Verification items for this drawing (mm, ordinates from the low corner). A direction names the side the tool comes from. Round coordinates to 2 decimals unless told otherwise and drop trailing zeros. Loops run counter-clockwise (first coordinate to the right, second up) from the corner with the lowest first, then second, coordinate; pieces in that order, holes last. Notation, with made-up numbers: (20, -7) - (36, -7) arc R10 ccw to (36, 12) - close; hole circle Ø10 at (59.25, 77). An arc over 180 degrees is marked (long way). Use a Markdown table: item, result. Add a question column.
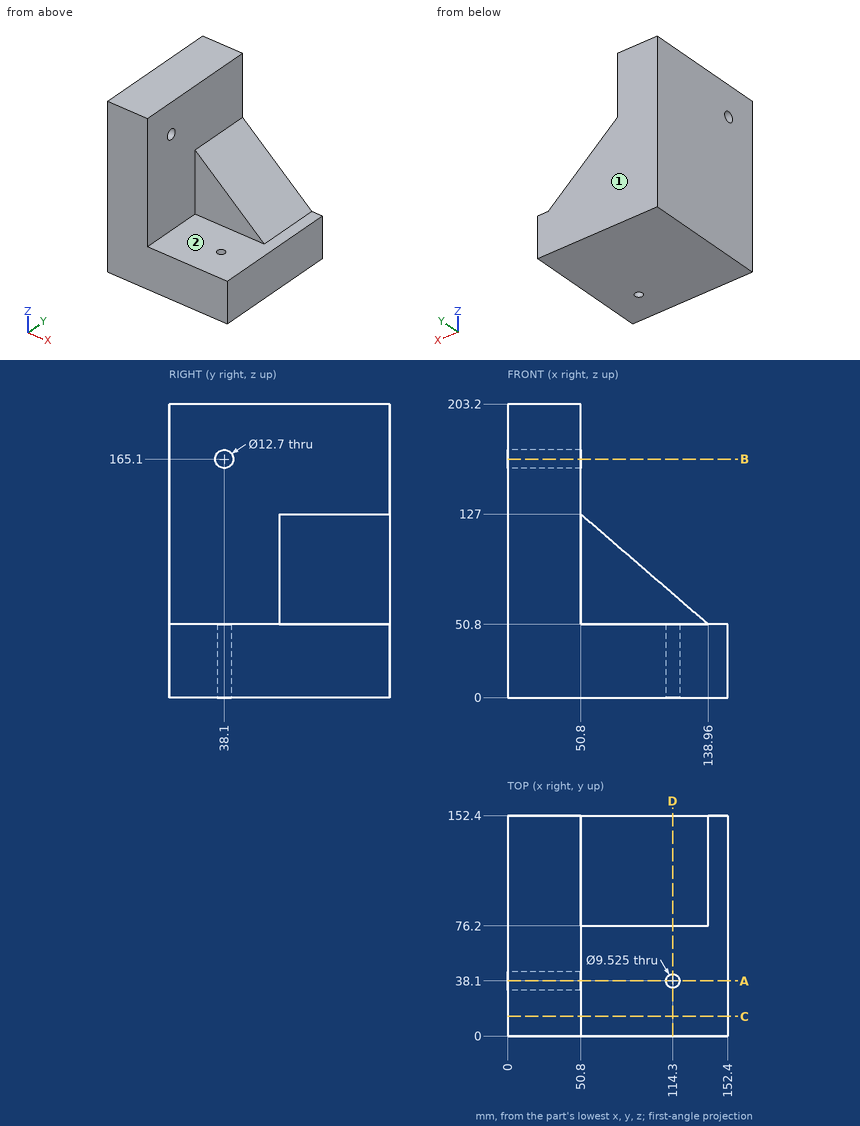
Q1. Section check D-D on x = 114.3. Record the cut outline in (y, z), plus the area to 3 significant figures.
Q2. Go/stop test with flat-tipped pins: pin 1 Ø5 at (y, z) = (36.5, 58.5) entering from +X; pin 2 Ø3 at (x, z) = (98.5, 77.5) entering from -Y. Record where each tip stops, or that it passes through.
Q3. Section check B-B on z = 165.1. Record the cut outline in (x, y).
Q4. Thickness scan on line 1 along Y through (x, z) = (18, 165); line 2 along Z through (x, y) = (31, 38); line 3 along Y through (x, z) = (114.3, 26.5). Record the ranges inside material, lowest first.
Q5. Section check C-C on y = 13.5. Record the cut outline in (x, z).
Q6. Set-up check for the marked faces 1 and 2: record each of +Z, -Z, +X, -X, +Y, -Y from which the full face is reachable in a straight line by a thin tool's end or side.
Q7. Section check A-A on y = 38.1. Record the cut outline in (x, z).
Determined:
| question | item | result |
|---|---|---|
| 1 | outline | (0, 0) - (33.34, 0) - (33.34, 50.8) - (0, 50.8) - close; (42.86, 0) - (152.4, 0) - (152.4, 72.11) - (76.2, 72.11) - (76.2, 50.8) - (42.86, 50.8) - close |
| 1 | area | 8,880 mm² |
| 2 | pin 1 | stops at x = 50.8 |
| 2 | pin 2 | stops at y = 76.2 |
| 3 | outline | (0, 0) - (50.8, 0) - (50.8, 31.75) - (0, 31.75) - close; (0, 44.45) - (50.8, 44.45) - (50.8, 152.4) - (0, 152.4) - close |
| 4 | line 1 | y = 0 to 31.75, 44.45 to 152.4 |
| 4 | line 2 | z = 0 to 158.75, 171.45 to 203.2 |
| 4 | line 3 | y = 0 to 33.34, 42.86 to 152.4 |
| 5 | outline | (0, 0) - (152.4, 0) - (152.4, 50.8) - (50.8, 50.8) - (50.8, 203.2) - (0, 203.2) - close |
| 6 | face 1 | +Z, -Z, +X, -X, +Y |
| 6 | face 2 | +Z, +X, -Y |
| 7 | outline | (0, 0) - (109.54, 0) - (109.54, 50.8) - (50.8, 50.8) - (50.8, 158.75) - (0, 158.75) - close; (0, 171.45) - (50.8, 171.45) - (50.8, 203.2) - (0, 203.2) - close; (119.06, 0) - (152.4, 0) - (152.4, 50.8) - (119.06, 50.8) - close |
